Geometry check sheet. Reference: the model listing, model coordinates, mm. Face numbers are marked on the shaded views. Round coordinates to 2 decimals unless told otherwise and drop trailing zeros. Order: outer loops, then holes, each group sorted by start corner. A loop starts at its lowest first (then second) coordinate and runs counter-clockwise, first axis right, second up.
(1) Draft check along X on the marked faces 1, 2 and 3. Enter one of: pulls with the +X half, pulls with the -X half, needs draft (parallel to the pull), parting line crosses it, or undercut.
(2) Gauge pin test, flat end, axial feed: P1, Ø3, axis at x = 11.67, y = -11.67, coming from the -Z side. Record the tip position at first contact, or that the pin passes through.
(3) Thickness scan on L1, parallel to Y at x = 0, z = 7; L2, parallel to X at y = 13, z = 7.5; L3, parallel to X at y = 12.5, z = 6.5. Record the ranges inside material, lowest first.
(4) Cross-section at A-A on x = 0. Enter the section's corners in (y, z), and give its area (3 significant figures).
(5) Cross-section at C-C on z = 6.25. Enter the section's corners in (x, y), and give its area (3 significant figures).
from build123d import *

# Parameters (mm, degrees)
SKETCH2_W             = 33.02
SKETCH2_H             = 33.02
BOSS_EXTRUDE1_DEPTH   = 12.7
SKETCH3_R             = 12.10437
CUT_EXTRUDE1_DEPTH    = 27.579130911
F_8_32_TAPPED_HOLE1_D = 3.4544
SKETCH9_R             = 12.7
CUT_EXTRUDE2_DEPTH    = 0.508


with BuildPart() as part:
    # Sketch2 → Boss-Extrude1 (new body)
    with BuildSketch(Plane.XY):
        Rectangle(SKETCH2_W, SKETCH2_H)
    extrude(amount=BOSS_EXTRUDE1_DEPTH)

    # Sketch3 → Cut-Extrude1 (cut, through all)
    with BuildSketch(Plane.XY.offset(12.7)):
        Circle(SKETCH3_R)
    extrude(amount=-CUT_EXTRUDE1_DEPTH, mode=Mode.SUBTRACT)

    # #8-32 Tapped Hole1 (through all)
    with Locations(Plane.XY.offset(12.7)):
        with Locations((-11.674332957, 11.674332957), (11.674332957, 11.674332957), (11.674332957, -11.674332957), (-11.674332957, -11.674332957)):
            Hole(F_8_32_TAPPED_HOLE1_D / 2)

    # Sketch9 → Cut-Extrude2 (cut)
    with BuildSketch(Plane(origin=(0, 0, 0), x_dir=(-1, 0, 0), z_dir=(0, 0, -1))):
        Circle(SKETCH9_R)
    extrude(amount=-CUT_EXTRUDE2_DEPTH, mode=Mode.SUBTRACT)


solid = part.part
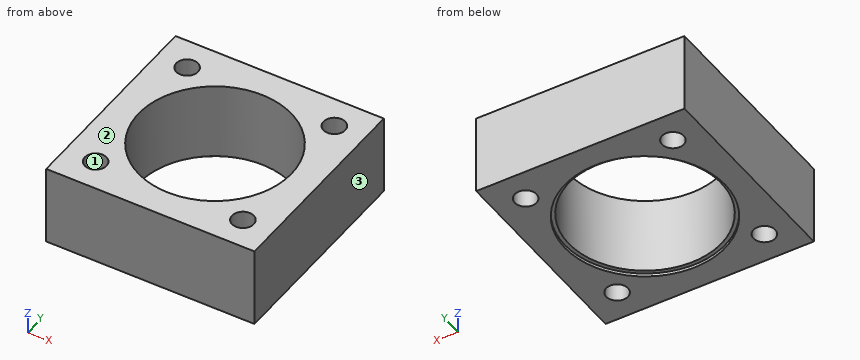
Found:
1. face 1: undercut
1. face 2: needs draft
1. face 3: pulls with the +X half
2. P1: passes through
3. L1: y = -16.51 to -12.1, 12.1 to 16.51
3. L2: x = -16.51 to -12.78, -10.57 to 10.57, 12.78 to 16.51
3. L3: x = -16.51 to -13.19, -10.16 to 10.16, 13.19 to 16.51
4. outline: (-16.51, 0) - (-12.7, 0) - (-12.7, 0.51) - (-12.1, 0.51) - (-12.1, 12.7) - (-16.51, 12.7) - close; (12.1, 0.51) - (12.7, 0.51) - (12.7, 0) - (16.51, 0) - (16.51, 12.7) - (12.1, 12.7) - close
4. area: 111 mm2
5. outline: (-16.51, -16.51) - (16.51, -16.51) - (16.51, 16.51) - (-16.51, 16.51) - close; hole circle Ø3.45 at (-11.67, -11.67); hole circle Ø3.45 at (-11.67, 11.67); hole circle Ø24.21 at (0, 0); hole circle Ø3.45 at (11.67, -11.67); hole circle Ø3.45 at (11.67, 11.67)
5. area: 593 mm2
